Geometry: final body of the model. Coordinates: model frame, mm. Face numbers are marked on the shaded views. A direction names the side the tool comes from. Round coordinates to 2 decimals unless told otherwise and drop trailing zeros. Loops run counter-clockwise (first coordinate to the right, second up) from the corner with the lowest first, then second, coordinate; pieces in that order, holes last. Notation, with made-up numbers: (60, 18.5) - (86, 18.5) arc R15 cw to (86, 47.5) - close; hole circle Ø8 at (27.25, -15.5). An arc over 180 degrees is marked (long way). Write item = value, one per line. Start each with the question number.
Item 1: Section B-B (y = 76.2). Return loops of the section in (x, z).
Item 2: Line query: line 1 (Y direction, x = -93.5, z = 0); line 2 (X direction, y = 129, z = 62); line 3 (Y direction, x = -5, z = 19.5). Output: solid intervals per line, ascending. Write a range as from..to.
Item 3: Section D-D (y = 105). Return loops of the section in (x, z), plus the area to 3 significant figures.
Item 4: First-contact query: pin 1 (1 mm diameter, centred on x = 81, z = -6.5, fed in from +Y); pin 2 (12 mm diameter, centred on x = 19.5, y = 109, fed in from -Z). Flat tips, straight axial feed; report the tip coordinate or a pass-through.
Item 5: Section A-A (z = 0). Return loops of the section in (x, y).
Item 6: Section C-C (x = 0). Return loops of the section in (y, z).
Item 7: Access query for the marked faces 4 and 5. Directions: +Z, -Z, +X, -X, +Y, -Y. A direction counts if a zero-diameter tool reaches every point of the face in a straight line with its end or side. Return the directions, or none.
Item 8: Draft query along X for the marked faces 1, 2 and 3. Return one class per face: pulls with the +X half, pulls with the -X half, needs draft (parallel to the pull), parting line crosses it, or undercut.
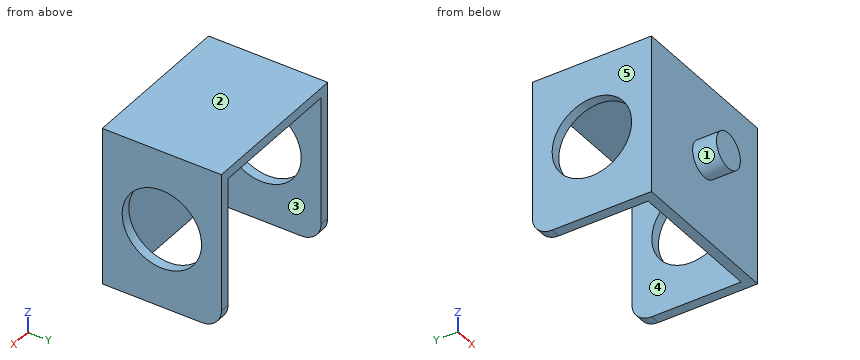
from build123d import *

# Parameters (mm, degrees)
SKETCH1_R           = 101.6
BOSS_EXTRUDE1_DEPTH = 152.4
SHELL1_T            = -12.7
SKETCH2_R           = 22.86
BOSS_EXTRUDE2_DEPTH = 30.48
SKETCH3_R           = 50.8
CUT_EXTRUDE1_DEPTH  = 274.566372202
FILLET1_R           = 25.4
FILLET2_R           = 25.4


with BuildPart() as part:
    # Sketch1 → Boss-Extrude1 (new body)
    with BuildSketch(Plane(origin=(0, 0, 0), x_dir=(1, 0, 0), z_dir=(0, 1, 0))):
        with BuildLine():
            ThreePointArc((101.6, 0), (71.842048938, -71.842048999), (-8.6e-08, -101.6))
            Line((-8.6e-08, -101.6), (101.6, -101.6))
            Line((101.6, -101.6), (101.6, 0))
        make_face()
        with BuildLine():
            ThreePointArc((-7e-08, 101.6), (71.842048944, 71.842048993), (101.6, 0))
            Line((101.6, 0), (101.6, 101.6))
            Line((101.6, 101.6), (-7e-08, 101.6))
        make_face()
        with BuildLine():
            Line((-101.6, 101.6), (-101.6, 8e-08))
            ThreePointArc((-101.6, 8e-08), (-71.842048965, 71.842048972), (-7e-08, 101.6))
            Line((-7e-08, 101.6), (-101.6, 101.6))
        make_face()
        with BuildLine():
            Line((-101.6, 8e-08), (-101.6, -101.6))
            Line((-101.6, -101.6), (-8.6e-08, -101.6))
            ThreePointArc((-8.6e-08, -101.6), (-71.842049028, -71.84204891), (-101.6, 8e-08))
        make_face()
        Circle(SKETCH1_R)
    extrude(amount=BOSS_EXTRUDE1_DEPTH)

    # Shell1
    shell1_openings = [part.faces().sort_by_distance(p)[0] for p in [
        (0, 152.4, 0),
        (0, 76.2, -101.6),
    ]]
    offset(amount=SHELL1_T, openings=shell1_openings, kind=Kind.INTERSECTION)

    # Sketch2 → Boss-Extrude2 (add)
    with BuildSketch(Plane.XZ):
        with Locations(Location((0, 0, 0), (0, 0, 90))):
            Circle(SKETCH2_R)
    extrude(amount=BOSS_EXTRUDE2_DEPTH)

    # Sketch3 → Cut-Extrude1 (cut, through all)
    with BuildSketch(Plane.ZY.offset(101.6)):
        with Locations((0, 76.2)):
            Circle(SKETCH3_R)
    extrude(amount=-CUT_EXTRUDE1_DEPTH, mode=Mode.SUBTRACT)

    # Fillet1
    fillet1_edges = [part.edges().sort_by_distance(p)[0] for p in [
        (-95.25, 152.4, -101.6),
    ]]
    fillet(fillet1_edges, radius=FILLET1_R)

    # Fillet2
    fillet2_edges = [part.edges().sort_by_distance(p)[0] for p in [
        (95.25, 152.4, -101.6),
    ]]
    fillet(fillet2_edges, radius=FILLET2_R)


solid = part.part
Taken from the geometry:
q1.outline = (-101.6, -101.6) - (-88.9, -101.6) - (-88.9, -50.8) - (-101.6, -50.8) - close; (-101.6, 50.8) - (-88.9, 50.8) - (-88.9, 88.9) - (88.9, 88.9) - (88.9, 50.8) - (101.6, 50.8) - (101.6, 101.6) - (-101.6, 101.6) - close; (88.9, -101.6) - (101.6, -101.6) - (101.6, -50.8) - (88.9, -50.8) - close
q2.line_1 = 0..25.4, 127..152.4
q2.line_2 = -101.6..-88.9, 88.9..101.6
q2.line_3 = -30.48..12.7
q3.outline = (-101.6, -101.6) - (-88.9, -101.6) - (-88.9, -41.85) - (-101.6, -41.85) - close; (-101.6, 41.85) - (-88.9, 41.85) - (-88.9, 88.9) - (88.9, 88.9) - (88.9, 41.85) - (101.6, 41.85) - (101.6, 101.6) - (-101.6, 101.6) - close; (88.9, -101.6) - (101.6, -101.6) - (101.6, -41.85) - (88.9, -41.85) - close
q3.area = 5,290 mm^2
q4.pin_1 = 12.7
q4.pin_2 = 88.9
q5.outline = (-101.6, 0) - (-22.86, 0) - (-22.86, -30.48) - (22.86, -30.48) - (22.86, 0) - (101.6, 0) - (101.6, 25.4) - (88.9, 25.4) - (88.9, 12.7) - (-88.9, 12.7) - (-88.9, 25.4) - (-101.6, 25.4) - close; (-101.6, 127) - (-88.9, 127) - (-88.9, 152.4) - (-101.6, 152.4) - close; (88.9, 127) - (101.6, 127) - (101.6, 152.4) - (88.9, 152.4) - close
q6.outline = (-30.48, -22.86) - (0, -22.86) - (0, -101.6) - (12.7, -101.6) - (12.7, 88.9) - (152.4, 88.9) - (152.4, 101.6) - (0, 101.6) - (0, 22.86) - (-30.48, 22.86) - close
q7.face_4 = -Z, +Y
q7.face_5 = +Z, -Z, -X, +Y, -Y
q8.face_1 = parting line crosses it
q8.face_2 = needs draft
q8.face_3 = undercut
